from build123d import *

# Parameters (mm, degrees)
ESQUISSE1_R        = 5
ESQUISSE1_R_2      = 1.05
BOSS_EXTRU_1_DEPTH = 2


with BuildPart() as part:
    # Esquisse1 → Boss.-Extru.1 (new body)
    with BuildSketch(Plane.XY):
        with BuildLine():
            Line((-7.996773354, 7.55325201), (-1.8, 8.818163074))
            ThreePointArc((-1.8, 8.818163074), (5.30110237, 7.27312269), (8.945833333, 0.985934061))
            ThreePointArc((8.945833333, 0.985934061), (9.25, 0), (8.945833333, -0.985934061))
            ThreePointArc((8.945833333, -0.985934061), (5.30110237, -7.27312269), (-1.8, -8.818163074))
            Line((-1.8, -8.818163074), (-7.996773354, -7.55325201))
            ThreePointArc((-7.996773354, -7.55325201), (-11, 0), (-7.996773354, 7.55325201))
        make_face()
        Circle(ESQUISSE1_R, mode=Mode.SUBTRACT)
        with Locations((7.5, 0)):
            Circle(ESQUISSE1_R_2, mode=Mode.SUBTRACT)
        with Locations((-6.01040764, 6.01040764)):
            Circle(ESQUISSE1_R_2, mode=Mode.SUBTRACT)
        with Locations(Location((-6.01040764, -6.01040764, 0), (0, 0, 180))):
            Circle(ESQUISSE1_R_2, mode=Mode.SUBTRACT)
    extrude(amount=BOSS_EXTRU_1_DEPTH)


solid = part.part
Work out the finished part from the listing and answer in its coordinate system (mm). Give positions to 0.01 mm unless a question says otherwise; leave off trailing zeros. Order: outer loops, then holes, each group sorted by start corner. A loop starts at its lowest first (then second) coordinate and runs counter-clockwise, first axis right, second up. Notation, with made-up numbers: M 78,23 L 118,23 A30 cw 118,62 Z; hole C -22,-34.5 d1. An arc over 180 degrees is marked long. Return JSON: item names as keys, results as strings.
Q1. This flat-tipped pin is pushed along its axis until it touches: pin 1 (1 mm diameter, centred on y = 6, z = 1, fed in from +X). Where does it stop, or does it pass through?
Answer below:
{"pin 1": "stops at x = 7.12"}
Q2. Find section B-B, the plane x = 0. Write down the section's boundary in (y, z).
Answer below:
{"outline": "M -9,0 L -5,0 L -5,2 L -9,2 Z; M 5,0 L 9,0 L 9,2 L 5,2 Z"}
Q3. The mould has two halves that part along Y. Classify faces 1 (the face through (-5.2, 0.1, 0)), 2 (the face through (-6.98, -5.61, 0.99)), 3 (the face through (5.4, -7.2, 1)): pulls with the +Y half, pulls with the -Y half, needs draft (parallel to the pull), parting line crosses it, or undercut.
Answer below:
{"face 1": "needs draft", "face 2": "undercut", "face 3": "pulls with the -Y half"}
Q4. Find section C-C, the plane z = 0.45. Write down the section's boundary in (x, y).
Answer below:
{"outline": "M -8,-7.55 L -1.8,-8.82 A9 ccw 8.95,-0.99 A1.75 ccw 8.95,0.99 A9 ccw -1.8,8.82 L -8,7.55 A11 ccw Z; hole C -6.01,-6.01 d2.1; hole C -6.01,6.01 d2.1; hole C 0,0 d10; hole C 7.5,0 d2.1"}
Q5. Find the intervals of material crossed by line 1 along Y through (x, z) = (0, 0.5); line 2 along Y through (x, z) = (1, 0.55); line 3 along X through (y, z) = (-4.25, 1.8), in increasing order. Write a range as [from, to].
Answer below:
{"line 1": "y = [-9, -5], [5, 9]", "line 2": "y = [-8.94, -4.9], [4.9, 8.94]", "line 3": "x = [-10.15, -2.63], [2.63, 7.93]"}
Q6. Find section A-A, the plane y = 0. Write down the section's boundary in (x, z).
Answer below:
{"outline": "M -11,0 L -5,0 L -5,2 L -11,2 Z; M 5,0 L 6.45,0 L 6.45,2 L 5,2 Z; M 8.55,0 L 9.25,0 L 9.25,2 L 8.55,2 Z"}
Q7. Find section D-D, the plane y = -2.75. Write down the section's boundary in (x, z).
Answer below:
{"outline": "M -10.65,0 L -4.18,0 L -4.18,2 L -10.65,2 Z; M 4.18,0 L 8.57,0 L 8.57,2 L 4.18,2 Z"}
